For this review, use the dimensioned drawing (mm, ordinates from the lowest corner) and the shaded views. Give positions to 0.01 mm unless a question says otherwise; leave off trailing zeros. Write each loop counter-clockwise with the first axis right and the second up, starting at its lowest first coordinate (ties: lowest second). Pieces come first, ordered by that corner, then holes. Notation, with made-up numbers: M 78,82.25 L 103,82.25 A30 cw 103,112.25 Z; hole C -11.75,-35.75 d2. An arc over 180 degrees is marked long. Answer in a Markdown table with one row per item.
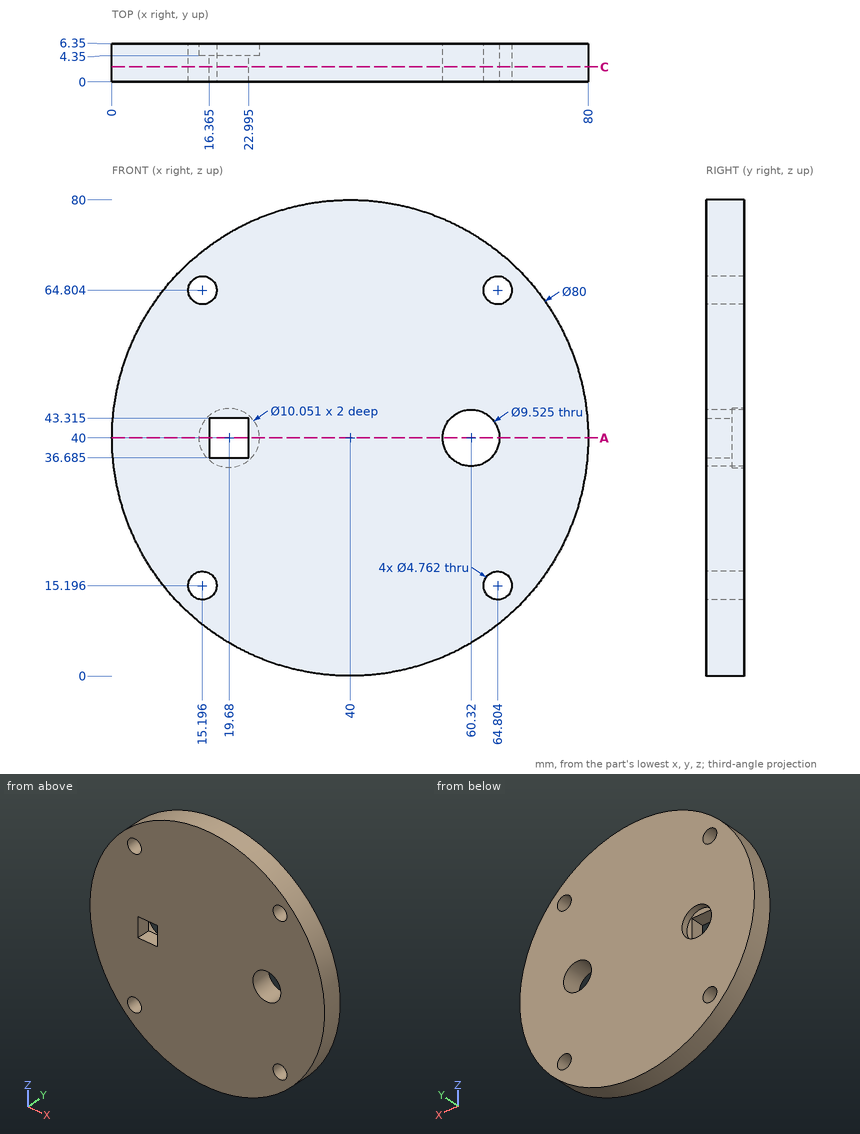
1) Add section C-C (y = 2.5). Write out the cut boundary in (x, z) (1 decimal).
Geometry says:
| item | result |
|---|---|
| outline | C 40,40 d80; hole C 15.2,15.2 d4.8; hole C 15.2,64.8 d4.8; hole M 16.4,36.7 L 23,36.7 L 23,43.3 L 16.4,43.3 Z; hole C 60.3,40 d9.5; hole C 64.8,15.2 d4.8; hole C 64.8,64.8 d4.8 |
2) Add section A-A (z = 40). Count the separate pieces of the cut face and the enclosed holes in it.
Geometry says:
| item | result |
|---|---|
| separate pieces | 3 |
| enclosed holes | 0 |
3) Insertion check: P1, Ø6, axis at x = 19.68, z = 40, coming from the +Y side; P2, Ø2, axis at x = 19, y = 2.5, coming from the -Z side; P3, Ø3.5, axis at y = 1.5, z = 41.5, coming from the -X side; P4, Ø3, axis at x = 26, y = 1.5, coming from the +Z side. Each pin has a flat end and moves straight along its axis. Give the tip position at first contact, or say it passes through.
Geometry says:
| item | result |
|---|---|
| P1 | through |
| P2 | z = 5.36 |
| P3 | x = 0 |
| P4 | z = 78 |
4) To check wall thickness, follow probe 1 along X at (y, z) = (4.75, 64) (1 decimal); probe 2 along X at (y, z) = (5.5, 44) (1 decimal); probe 3 along Z at (x, y) = (60.32, 4.25) (1 decimal). State the ranges of each line that lie inside material, in increasing order. Write a range as [from, to].
Geometry says:
| item | result |
|---|---|
| probe 1 | [8, 13], [17.4, 62.6], [67, 72] |
| probe 2 | [0.2, 16.6], [22.7, 57.7], [62.9, 79.8] |
| probe 3 | [5.5, 35.2], [44.8, 74.5] |
